Source: CAD feature listing. Evaluate the final solid. Frame: model axes, mm. Face numbers are marked on the shaded views. A direction names the side the tool comes from. Give positions to 0.01 mm unless a question says otherwise; leave off trailing zeros. Write each loop counter-clockwise with the first axis right and the second up, starting at its lowest first coordinate (ties: lowest second). Pieces come first, ordered by that corner, then holes. Notation, with made-up numbers: M 9.5,44 L 46.5,44 A23 cw 46.5,79 Z; hole C 2.5,32 d10. An arc over 180 degrees is marked long. Answer as a JSON object with one key per item and string values. Group by question number.
```python
from build123d import *

# Parameters (mm, degrees)
SKETCH1_R               = 2.5
BOSS_EXTRUDE1_DEPTH     = 5
SKETCH4_R               = 1.5
CUT_EXTRUDE1_DEPTH      = 10.988857319
SKETCH5_W               = 10.682767576
SKETCH5_H               = 3.673973587
CUT_EXTRUDE2_DEPTH      = 4.5
CUT_EXTRUDE2_DEPTH_BACK = 4.5
CHAMFER1_SIZE           = 1


with BuildPart() as part:
    # Sketch1 → Boss-Extrude1 (new body)
    with BuildSketch(Plane.XY):
        with BuildLine():
            Line((-20.645898034, 1), (-3.354101966, 1))
            ThreePointArc((-3.354101966, 1), (3.5, 0), (-3.354101966, -1))
            Line((-3.354101966, -1), (-20.645898034, -1))
            ThreePointArc((-20.645898034, -1), (-27.5, 0), (-20.645898034, 1))
        make_face()
        Circle(SKETCH1_R, mode=Mode.SUBTRACT)
        with Locations((-24, 0)):
            Circle(SKETCH1_R, mode=Mode.SUBTRACT)
    extrude(amount=BOSS_EXTRUDE1_DEPTH)

    # Sketch3 → Revolve1 (revolve)
    with BuildSketch(Plane(origin=(0, 0, 0), x_dir=(1, 0, 0), z_dir=(0, 1, 0))):
        Polygon((-8.70524893, 1.372812946), (-7.43068634, -5), (-10.862718705, -5.686406473), (-12.137281295, 0.686406473), align=None)
    revolve(axis=Axis((-12.027607656, 0, -0.138038281), (0.196116135, 0, 0.980580676)))

    # Sketch4 → Cut-Extrude1 (cut, through all)
    with BuildSketch(Plane(origin=(-0.598819756, 0, -2.994098781), x_dir=(-0.980580676, 0, 0.196116135), z_dir=(-0.196116135, 0, -0.980580676))):
        with Locations((11.766968108, 0)):
            Circle(SKETCH4_R)
    extrude(amount=-CUT_EXTRUDE1_DEPTH, mode=Mode.SUBTRACT)

    # Sketch5 → Cut-Extrude2 (cut, two sides)
    with BuildSketch(Plane(origin=(0, 0, 0), x_dir=(1, 0, 0), z_dir=(0, 1, 0))) as cut_extrude2_sk:
        with Locations((-12.153708886, 1.836986794)):
            Rectangle(SKETCH5_W, SKETCH5_H)
    extrude(amount=CUT_EXTRUDE2_DEPTH, mode=Mode.SUBTRACT)
    extrude(cut_extrude2_sk.sketch, amount=-CUT_EXTRUDE2_DEPTH_BACK, mode=Mode.SUBTRACT)

    # Chamfer1
    chamfer1_edges = [part.edges().sort_by_distance(p)[0] for p in [
        (-9.391847692, 0, 5.39223227),
    ]]
    chamfer(chamfer1_edges, length=CHAMFER1_SIZE)


solid = part.part
```
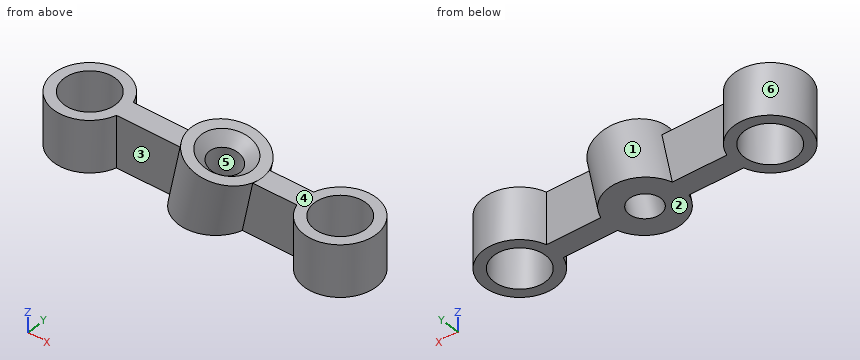
(1) Pull-direction query (Y, two-part tool) for the marked faces 4, 5 and 6; classes: pulls with the +Y half, pulls with the -Y half, needs draft (parallel to the pull), parting line crosses it, or undercut.
(2) Ray query, L1, parallel to Y at x = 0, z = 2.9; L2, parallel to X at y = 3, z = 1; L3, parallel to X at y = -2.75, z = 3. Return the intervals inside material, ascending. Write a range as [from, to].
(3) Contact query for flat-ended pins moving along their axis: pin 1 Ø2 at (x, z) = (-1, 4) entering from -Y; pin 2 Ø2.5 at (x, z) = (-6, 3) entering from +Y; pin 3 Ø2.5 at (x, z) = (-6.5, 2.5) entering from -Y. Output: stop coordinate, or through.
(4) Section B-B, the plane z = 1. State how many separate pieces and enclosed holes the cut face has, plus the area to 3 significant figures.
(5) Access query for the marked faces 1, 2 and 3. Directions: +Z, -Z, +X, -X, +Y, -Y. A direction counts if a zero-diameter tool reaches every point of the face in a straight line with its end or side. Return the directions, or none.
(6) Section A-A, the plane x = 0. Return loops of the section in (y, z).
Reported:
{
 "1": {"face 4": "needs draft", "face 5": "undercut", "face 6": "parting line crosses it"},
 "2": {"L1": "y = [-3.5, -2.5], [2.5, 3.5]", "L2": "x = [-25.8, -22.2], [-13.64, -9.96], [-1.8, 1.8]", "L3": "x = [-26.17, -21.83], [-13.61, -9.19], [-2.17, 2.17]"},
 "3": {"pin 1": "stops at y = -3.5", "pin 2": "stops at y = 1", "pin 3": "stops at y = -1"},
 "4": {"separate pieces": "1", "enclosed holes": "3", "area": "89.8 mm2"},
 "5": {"face 1": "none", "face 2": "-Z, +X, -X, +Y, -Y", "face 3": "+Z, -Y"},
 "6": {"outline": "M -3.5,0 L -2.5,0 L -2.5,5 L -3.5,5 Z; M 2.5,0 L 3.5,0 L 3.5,5 L 2.5,5 Z"}
}
